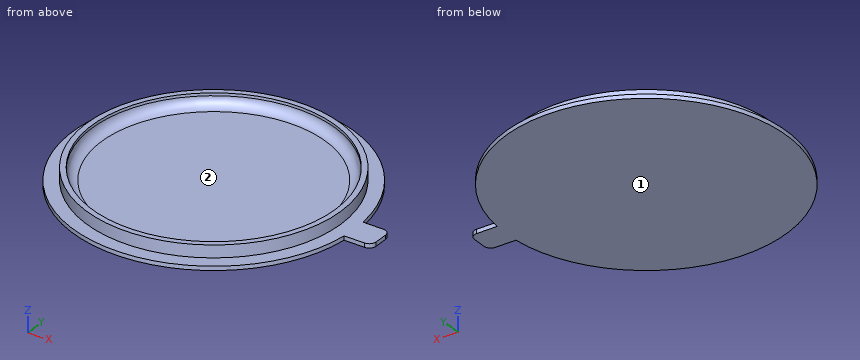
from build123d import *

# Parameters (mm, degrees)
F0_R     = 93
F0_R_2   = 89
F1_DEPTH = 3
F2_DEPTH = 12
F3_R     = 7


with BuildPart() as f1:
    # F0 (on Top) → F1 (new body)
    with BuildSketch(Plane.XY):
        with BuildLine():
            ThreePointArc((102.5134137564, -10), (102.8782815197, -5.0059156548), (103, 0))
            ThreePointArc((103, 0), (102.8782815197, 5.0059156548), (102.5134137564, 10))
            ThreePointArc((102.5134137564, 10), (-103, 0), (102.5134137564, -10))
        make_face()
        Circle(F0_R, mode=Mode.SUBTRACT)
        Circle(F0_R)
        Circle(F0_R_2, mode=Mode.SUBTRACT)
        Circle(F0_R_2)
        with BuildLine():
            ThreePointArc((102.5134137564, 10), (102.8782815197, 5.0059156548), (103, 0))
            ThreePointArc((103, 0), (102.8782815197, -5.0059156548), (102.5134137564, -10))
            Line((102.5134137564, -10), (117.5134137564, -10))
            ThreePointArc((117.5134137564, -10), (121.0489476624, -8.5355339059), (122.5134137564, -5))
            Line((122.5134137564, -5), (122.5134137564, 0))
            Line((122.5134137564, 0), (122.5134137564, 5))
            ThreePointArc((122.5134137564, 5), (121.0489476624, 8.5355339059), (117.5134137564, 10))
            Line((117.5134137564, 10), (102.5134137564, 10))
        make_face()
    extrude(amount=F1_DEPTH)

    # F0 (on Top) → F2 (join)
    with BuildSketch(Plane.XY):
        Circle(F0_R)
        Circle(F0_R_2, mode=Mode.SUBTRACT)
    extrude(amount=F2_DEPTH)

    # F3
    f3_edges = [f1.edges().sort_by_distance(p)[0] for p in [
        (-89, 0, 3),
    ]]
    fillet(f3_edges, radius=F3_R)


solid = f1.part
The listing builds one solid part. Answer for the finished solid, in the listing's coordinates (mm). Face numbers are marked on the shaded views. Give positions to 0.01 mm unless a question says otherwise; leave off trailing zeros. Write each loop counter-clockwise with the first axis right and the second up, starting at its lowest first coordinate (ties: lowest second). Pieces come first, ordered by that corner, then holes.
1) Section C-C (z = 8) is taken. Write down the section's boundary in (x, y).
2) Section B-B (x = 0) is taken. Write down the section's boundary in (y, z), and give its area (3 significant figures).
3) For a pull along X with two mould halves and no side action, classify the marked faces 1 and 2 as pulls with the +X half, pulls with the -X half, needs draft (parallel to the pull), parting line crosses it, or undercut.
4) Find the intervals of material crossed by L1, parallel to X at y = 0, z = 11.6; L2, parallel to Y at x = 65, z = 8.5, in increasing order.
5) Given P1, Ø0.9, axis at x = 112.5, z = 2, coming from the +Y side; P2, Ø1.5, axis at y = 71.5, z = 9.5, coming from the +X side; P3, Ø12, axis at x = -77, y = -5, coming from the +Z side, each flat-ended and moving along its own axis, determine where each tip first touches the part or whether it passes through.
6) Section A-A (y = 0) is taken. Write down the section's boundary in (x, z), and give its area (3 significant figures).
Response:
1. outline: circle Ø186 at (0, 0); hole circle Ø177.42 at (0, 0)
2. outline: (-103, 0) - (103, 0) - (103, 3) - (93, 3) - (93, 12) - (89, 12) - (89, 10) arc R7 cw to (82, 3) - (-82, 3) arc R7 cw to (-89, 10) - (-89, 12) - (-93, 12) - (-93, 3) - (-103, 3) - close
2. area: 711 mm2
3. face 1: needs draft
3. face 2: undercut
4. L1: x = -93 to -89, 89 to 93
4. L2: y = -66.51 to -60.56, 60.56 to 66.51
5. P1: stops at y = 10
5. P2: stops at x = 60.36
5. P3: stops at z = 3.1
6. outline: (-103, 0) - (122.51, 0) - (122.51, 3) - (93, 3) - (93, 12) - (89, 12) - (89, 10) arc R7 cw to (82, 3) - (-82, 3) arc R7 cw to (-89, 10) - (-89, 12) - (-93, 12) - (-93, 3) - (-103, 3) - close
6. area: 770 mm2
